from build123d import *

# Parameters (mm, degrees)
SKETCH1_W           = 63.5
SKETCH1_H           = 100
SKETCH1_R           = 3.5
SKETCH1_R_2         = 10
BOSS_EXTRUDE1_DEPTH = 6.35


with BuildPart() as part:
    # Sketch1 → Boss-Extrude1 (new body)
    with BuildSketch(Plane.XY):
        with Locations((0, 50)):
            Rectangle(SKETCH1_W, SKETCH1_H)
        with Locations((-19.05, 12.7)):
            Circle(SKETCH1_R, mode=Mode.SUBTRACT)
        with Locations(Location((-19.05, 87.3, 0), (0, 0, 180))):
            Circle(SKETCH1_R, mode=Mode.SUBTRACT)
        with Locations((12.7, 50)):
            Circle(SKETCH1_R_2, mode=Mode.SUBTRACT)
    extrude(amount=BOSS_EXTRUDE1_DEPTH)


solid = part.part
The model under review builds one solid part; all positions refer to its coordinate system, in mm. Round coordinates to 2 decimals unless told otherwise and drop trailing zeros. Order: outer loops, then holes, each group sorted by start corner. A loop starts at its lowest first (then second) coordinate and runs counter-clockwise, first axis right, second up. Notation, with made-up numbers: (-8, 22.5) -> (-1, 22.5) arc R14 ccw to (-1, 28.5) -> close; hole circle Ø7 at (28, 20). An arc over 180 degrees is marked (long way). Use CSV: the item, a comma, the result in double quotes. Start each with the question number.
(1) Wall thickness on probe 1 along Y at (x, z) = (-19.05, 2.5); probe 2 along Y at (x, z) = (12.7, 2.75); probe 3 along Y at (x, z) = (-21, 6.25): over which ranges is each line inside the solid? List them lowest first. Write a range as from..to.
(2) Insertion check: pin 1 (12 mm diameter, centred on x = -14.5, y = 74, fed in from -Z). The pin has a flat end and moves straight along its axis. Give the tip position at first contact, or say it passes through.
(3) Consider section C-C on x = -19.05. Write out the cut boundary in (y, z).
(4) Mouldability with a two-part tool opening along X and no side actions: class faces 1 (the face through (31.75, 49, 3)), 2 (the face through (0, 51, 6.35)), 3 (the face through (-18.291, 90.717, 3.131)) as pulls with the +X half, pulls with the -X half, needs draft (parallel to the pull), parting line crosses it, or undercut.
(5) Consider section A-A on y = 12.7. Write out the cut boundary in (x, z), and give its area (3 significant figures).
(6) Consider section D-D on z = 4.5. Write out the cut boundary in (x, y), and give its area (3 significant figures).
(7) Consider section B-B on x = 12.7. Write out the cut boundary in (y, z), and give its area (3 significant figures).
Responses:
1,probe 1,"0..9.2, 16.2..83.8, 90.8..100"
1,probe 2,"0..40, 60..100"
1,probe 3,"0..9.79, 15.61..84.39, 90.21..100"
2,pin 1,"z = 0"
3,outline,"(0, 0) -> (9.2, 0) -> (9.2, 6.35) -> (0, 6.35) -> close; (16.2, 0) -> (83.8, 0) -> (83.8, 6.35) -> (16.2, 6.35) -> close; (90.8, 0) -> (100, 0) -> (100, 6.35) -> (90.8, 6.35) -> close"
4,face 1,"pulls with the +X half"
4,face 2,"needs draft"
4,face 3,"undercut"
5,outline,"(-31.75, 0) -> (-22.55, 0) -> (-22.55, 6.35) -> (-31.75, 6.35) -> close; (-15.55, 0) -> (31.75, 0) -> (31.75, 6.35) -> (-15.55, 6.35) -> close"
5,area,"359 mm²"
6,outline,"(-31.75, 0) -> (31.75, 0) -> (31.75, 100) -> (-31.75, 100) -> close; hole circle Ø7 at (-19.05, 12.7); hole circle Ø7 at (-19.05, 87.3); hole circle Ø20 at (12.7, 50)"
6,area,"5,960 mm²"
7,outline,"(0, 0) -> (40, 0) -> (40, 6.35) -> (0, 6.35) -> close; (60, 0) -> (100, 0) -> (100, 6.35) -> (60, 6.35) -> close"
7,area,"508 mm²"
